from build123d import *

# Parameters (mm, degrees)
BOSS_EXTRUDE2_DEPTH = 124
FILLET1_R           = 15
FILLET2_R           = 15
SKETCH2_W           = 60
SKETCH2_H           = 35
BOSS_EXTRUDE3_DEPTH = 27
SKETCH5_R           = 20
CUT_EXTRUDE8_DEPTH  = 50


with BuildPart() as part:
    # Sketch1 → Boss-Extrude2 (new body)
    with BuildSketch(Plane.XY):
        Polygon((0, 0), (60, 0), (60, 50), (45, 50), (45, 15), (0, 15), align=None)
    extrude(amount=BOSS_EXTRUDE2_DEPTH)

    # Fillet1
    fillet1_edges = [part.edges().sort_by_distance(p)[0] for p in [
        (52.5, 50, 124),
        (0, 7.5, 124),
        (52.5, 50, 0),
    ]]
    fillet(fillet1_edges, radius=FILLET1_R)

    # Fillet2
    fillet2_edges = [part.edges().sort_by_distance(p)[0] for p in [
        (0, 7.5, 0),
    ]]
    fillet(fillet2_edges, radius=FILLET2_R)

    # Sketch2 → Boss-Extrude3 (add)
    with BuildSketch(Plane.ZY.offset(-45)):
        with Locations((62, 32.5)):
            Rectangle(SKETCH2_W, SKETCH2_H)
    extrude(amount=BOSS_EXTRUDE3_DEPTH)

    # Sketch5 → Cut-Extrude8 (cut)
    with BuildSketch(Plane.ZY.offset(-18)):
        with Locations((62, 50)):
            Circle(SKETCH5_R)
    extrude(amount=-CUT_EXTRUDE8_DEPTH, mode=Mode.SUBTRACT)


solid = part.part
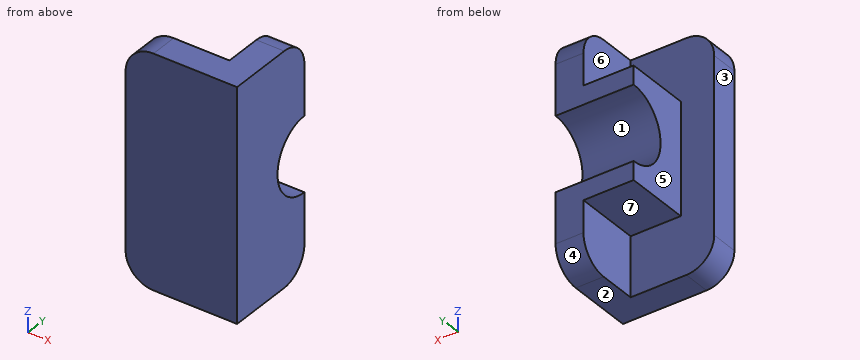
For this review, take the finished solid that the model builds, in its own axes (mm). Face numbers are marked on the shaded views. A direction names the side the tool comes from. Coordinates: 2 decimals unless noted, no trailing zeros. Order: outer loops, then holes, each group sorted by start corner. A loop starts at its lowest first (then second) coordinate and runs counter-clockwise, first axis right, second up. Notation, with made-up numbers: (-3.75, 31) -> (9.25, 31) arc R5 ccw to (9.25, 39) -> close; hole circle Ø9 at (-31, 71.25). An arc over 180 degrees is marked (long way). Return JSON: item names as keys, results as strings.
1. We need section C-C on z = 62. Write out the cut boundary in (x, y).
Answer block:
{"outline": "(0, 0) -> (60, 0) -> (60, 30) -> (18, 30) -> (18, 15) -> (0, 15) -> close"}
2. Machinability: for the marked faces 4, 5, 6 and 7, which of the approach directions +Z, -Z, +X, -X, +Y, -Y give a long, thin tool a straight path to every point of the face, cutting with its end or side? Answer none if there is none.
Answer block:
{"face 4": "-Z, +X, -X, +Y", "face 5": "+Z, -Z, -X, +Y", "face 6": "+Z, -X, +Y", "face 7": "-Z, -X, +Y"}
3. We need section D-D on y = 17. Write out the cut boundary in (x, z).
Answer block:
{"outline": "(18, 32) -> (45, 32) -> (45, 0) -> (60, 0) -> (60, 124) -> (45, 124) -> (45, 92) -> (18, 92) -> close"}
4. For pin 1 Ø6 at (x, z) = (16, 16) entering from +Y; pin 2 Ø4 at (x, y) = (28, 33) entering from -Z; pin 3 Ø1.5 at (x, y) = (16.5, 41.5) entering from -Z; pin 4 Ø13.5 at (x, y) = (25.5, 35.5) entering from +Z, all flat-tipped, find the tip position at first contact; note any pin that passes through.
Answer block:
{"pin 1": "y = 15", "pin 2": "z = 32", "pin 3": "through", "pin 4": "z = 92"}
5. The part is to be moulded in two halves that separate along Z. For the marked faces 1, 2 and 3, say which applies: +Z half, -Z half, draft (parallel to the pull), parting line (faces both ways), or undercut.
Answer block:
{"face 1": "undercut", "face 2": "-Z half", "face 3": "draft"}
6. We need section A-A on y = 37.5. Write out the cut boundary in (x, z).
Answer block:
{"outline": "(18, 32) -> (45, 32) -> (45, 0.21) -> (60, 0.21) -> (60, 46.39) -> (18, 46.39) -> close; (18, 77.61) -> (60, 77.61) -> (60, 123.79) -> (45, 123.79) -> (45, 92) -> (18, 92) -> close"}
7. We need section B-B on x = 35.5. Write out the cut boundary in (y, z), and give its area (3 significant figures).
Answer block:
{"outline": "(0, 0) -> (15, 0) -> (15, 32) -> (50, 32) -> (50, 42) arc R20 cw to (50, 82) -> (50, 92) -> (15, 92) -> (15, 124) -> (0, 124) -> close", "area": "3,330 mm²"}
8. For line 1 (Y direction, x = 12.5, z = 12.5); line 2 (X direction, y = 16.5, z = 115); line 3 (X direction, y = 31.5, z = 74.5), list the stretches that pass through material, from the lowest coordinate up. Write a range as from..to.
Answer block:
{"line 1": "0..15", "line 2": "45..60", "line 3": "18..60"}
